```python
from build123d import *

# Parameters (mm, degrees)
SKETCH1_W                    = 100
SKETCH1_H                    = 100
BOSS_EXTRUDE1_DEPTH          = 50
BOSS_EXTRUDE1_DRAFT          = -1
SKETCH3_W                    = 80
SKETCH3_H                    = 30
CUT_EXTRUDE2_DEPTH           = 15
FILLET1_R                    = 10
SKETCH4_R                    = 10
CUT_EXTRUDE3_DEPTH           = 15
CUT_EXTRUDE3_DRAFT           = -0.5
CUT_EXTRUDE3_PROFILE_2_DEPTH = 15
CUT_EXTRUDE3_PROFILE_2_DRAFT = -0.5
SKETCH5_R                    = 10
CUT_EXTRUDE4_DEPTH           = 30
FILLET2_R                    = 0.5


with BuildPart() as part:
    # Sketch1 → Boss-Extrude1 (with draft: the straight prism first)
    with BuildSketch(Plane(origin=(0, 0, 0), x_dir=(1, 0, 0), z_dir=(0, 1, 0))):
        with Locations((50, 50)):
            Rectangle(SKETCH1_W, SKETCH1_H)
    extrude(amount=BOSS_EXTRUDE1_DEPTH)
    # Boss-Extrude1: the draft: its side faces are tilted about the plane it starts from
    boss_extrude1_sides = [part.faces().sort_by_distance(p)[0] for p in [
        (50, 25, 0),
        (100, 25, -50),
        (50, 25, -100),
        (0, 25, -50),
    ]]
    draft(boss_extrude1_sides, Plane(origin=(0, 0, 0), x_dir=(1, 0, 0), z_dir=(0, 1, 0)), BOSS_EXTRUDE1_DRAFT)

    # Sketch3 → Cut-Extrude2 (cut)
    with BuildSketch(Plane(origin=(0, 50, 0), x_dir=(1, 0, 0), z_dir=(0, 1, 0))):
        with Locations((49.127246754, 24.127246754)):
            Rectangle(SKETCH3_W, SKETCH3_H)
    extrude(amount=-CUT_EXTRUDE2_DEPTH, mode=Mode.SUBTRACT)

    # Fillet1
    fillet1_edges = [part.edges().sort_by_distance(p)[0] for p in [
        (9.127246754, 42.5, -9.127246754),
        (9.127246754, 42.5, -39.127246754),
        (89.127246754, 42.5, -39.127246754),
        (89.127246754, 42.5, -9.127246754),
    ]]
    fillet(fillet1_edges, radius=FILLET1_R)


with BuildPart() as cut_extrude3_tool:
    # Sketch4 → Cut-Extrude3 (with draft: the straight prism first)
    with BuildSketch(Plane(origin=(0, 35, 0), x_dir=(1, 0, 0), z_dir=(0, 1, 0))):
        with Locations((24.127246754, 24.127246754)):
            Circle(SKETCH4_R)
    extrude(amount=-CUT_EXTRUDE3_DEPTH)
    # Cut-Extrude3: the draft: its side faces are tilted about the plane it starts from
    cut_extrude3_sides = [cut_extrude3_tool.faces().sort_by_distance(p)[0] for p in [
        (14.127246754, 27.5, -24.127246754),
    ]]
    draft(cut_extrude3_sides, Plane(origin=(0, 35, 0), x_dir=(1, 0, 0), z_dir=(0, 1, 0)), CUT_EXTRUDE3_DRAFT)


with BuildPart() as part_1:
    add(part.part)

    # Cut-Extrude3: cut by cut_extrude3_tool
    add(cut_extrude3_tool.part, mode=Mode.SUBTRACT)


with BuildPart() as cut_extrude3_profile_2_tool:
    # Sketch4 → Cut-Extrude3 profile 2 (with draft: the straight prism first)
    with BuildSketch(Plane(origin=(0, 35, 0), x_dir=(1, 0, 0), z_dir=(0, 1, 0))):
        with Locations((74.127246754, 24.127246754)):
            Circle(SKETCH4_R)
    extrude(amount=-CUT_EXTRUDE3_PROFILE_2_DEPTH)
    # Cut-Extrude3 profile 2: the draft: its side faces are tilted about the plane it starts from
    cut_extrude3_profile_2_sides = [cut_extrude3_profile_2_tool.faces().sort_by_distance(p)[0] for p in [
        (64.127246754, 27.5, -24.127246754),
    ]]
    draft(cut_extrude3_profile_2_sides, Plane(origin=(0, 35, 0), x_dir=(1, 0, 0), z_dir=(0, 1, 0)), CUT_EXTRUDE3_PROFILE_2_DRAFT)


with BuildPart() as part_2:
    add(part_1.part)

    # Cut-Extrude3 profile 2: cut by cut_extrude3_profile_2_tool
    add(cut_extrude3_profile_2_tool.part, mode=Mode.SUBTRACT)

    # Sketch5 → Cut-Extrude4 (cut)
    with BuildSketch(Plane(origin=(0, 35, 0), x_dir=(1, 0, 0), z_dir=(0, 1, 0))):
        with Locations(Location((49.127246754, 24.127246754, 0), (0, 0, 270))):
            Circle(SKETCH5_R)
    extrude(amount=-CUT_EXTRUDE4_DEPTH, mode=Mode.SUBTRACT)

    # Fillet2
    fillet2_edges = [part_2.edges().sort_by_distance(p)[0] for p in [
        (100.872753246, 50, -50),
        (50, 50, -100.872753246),
        (-0.872753246, 50, -50),
        (50, 0, -100),
        (100, 0, -50),
        (50, 0, 0),
        (0, 0, -50),
        (50, 50, 0.872753246),
        (-0.436376623, 25, -100.436376623),
        (100.436376623, 25, -100.436376623),
        (100.436376623, 25, 0.436376623),
        (-0.436376623, 25, 0.436376623),
    ]]
    fillet(fillet2_edges, radius=FILLET2_R)


solid = part_2.part
```
Input: part model. Units: mm. Frame: model coordinates. A direction names the side the tool comes from. Coordinates: 2 decimals unless noted, no trailing zeros. Loops run counter-clockwise (first coordinate to the right, second up) from the corner with the lowest first, then second, coordinate; pieces in that order, holes last.
Q1. Section B-B, the plane y = 29.5. Give the number of separate pieces and of enclosed holes in the cut face, and give its area (3 significant figures).
Results are:
separate pieces: 1
enclosed holes: 3
area: 9,270 mm2
Q2. Line query: line 1 along X through (y, z) = (24, -17); line 2 along X through (y, z) = (40, -31.5); line 3 along X through (y, z) = (20, -38). Output: solid intervals per line, ascending.
Results are:
line 1: x = -0.42 to 17.25, 31 to 42.11, 56.14 to 67.25, 81 to 100.42
line 2: x = -0.7 to 9.41, 88.84 to 100.7
line 3: x = -0.35 to 100.35
Q3. Section A-A, the plane z = -35.5. Return the cut outline in (x, y).
Results are:
outline: (-0.86, 49.49) - (-0.01, 0.49) arc R0.5 ccw to (0.49, 0) - (99.51, 0) arc R0.5 ccw to (100.01, 0.49) - (100.86, 49.49) arc R0.5 ccw to (100.36, 50) - (86.83, 50) - (86.83, 35) - (11.42, 35) - (11.42, 50) - (-0.36, 50) arc R0.5 ccw to start
Q4. Set-up query: faces 3 (the flat face through (24, 20, -24)), 4 (the flat face through (49, 50, -62)). Return all of +Z, -Z, +X, -X, +Y, -Y with unobstructed straight access to the full face (end or side cutting, diameter ignored); none if empty.
Results are:
face 3: +Y
face 4: +Z, -Z, +X, -X, +Y
Q5. Mould query, pull axis X, two halves, no side actions, for faces 1 (the cylindrical face through (12.134, 42.395, -36.276)), 2 (the flat face through (49, 0, -51)). Classes: +X half, -X half, draft (parallel to the pull), parting line (faces both ways), or undercut.
Results are:
face 1: undercut
face 2: draft
Q6. Contact query for flat-ended pins moving along their axis: pin 1 (1.5 mm diameter, centred on y = 40.5, z = -39.5, fed in from +X); pin 2 (3 mm diameter, centred on y = 46, z = -25, fed in from -X); pin 3 (8 mm diameter, centred on y = 20.5, z = -58, fed in from -X). Output: stop coordinate, or through.
Results are:
pin 1: stops at x = 100.72
pin 2: stops at x = -0.83
pin 3: stops at x = -0.43
